The figure shows three views and two pictorial views of one solid part (mm, origin at its lowest corner). Answer the questions. A direction names the side the tool comes from. Round coordinates to 2 decimals unless told otherwise and drop trailing zeros. Order: outer loops, then holes, each group sorted by start corner. A loop starts at its lowest first (then second) coordinate and runs counter-clockwise, first axis right, second up. Notation, with made-up numbers: (33, -16.5) -> (75, -16.5) arc R20 ccw to (75, 17.5) -> close; hole circle Ø4 at (38.5, 22.5). An arc over 180 degrees is marked (long way). Answer as a JSON object with one key per item and string values. Group by question number.
Item 1: Given P1, Ø6.5, axis at x = 19.5, y = 6, coming from the -Z side; P2, Ø3, axis at x = 118, z = 2.5, coming from the +Y side; P3, Ø10, axis at x = 71.5, z = 26, coming from the +Y side; P4, Ø18, axis at x = 57, y = 71.5, coming from the -Z side, each flat-ended and moving along its own axis, determine where each tip first touches the part or whether it passes through.
Item 2: The mould has two halves that part along Y. Classify the marked faces 6, 7 and 8: pulls with the +Y half, pulls with the -Y half, needs draft (parallel to the pull), parting line crosses it, or undercut.
Item 3: For the marked faces 1, 2, 3, 4 and 5, determine the directions among +Z, -Z, +X, -X, +Y, -Y from which every point of the face is accessible in a straight line to the end or side of a thin tool.
Item 4: Section D-D, the plane z = 16.5 is taken. Write down the section's boundary in (x, y).
Item 5: Section C-C, the plane y = 12 is taken. Write down the section's boundary in (x, z), plus the area to 3 significant figures.
Item 6: Consider probe 1 along Y at (x, z) = (65, 6.5); probe 2 along Z at (x, y) = (88, 68); probe 3 along X at (y, z) = (72, 6). Determine where each line is inside the solid, lowest interval first. Write a range as from..to.
Item 7: Section A-A, the plane x = 65 is taken. Write down the section's boundary in (y, z).
Item 8: Section B-B, the plane z = 37 is taken. Write down the section's boundary in (x, y).
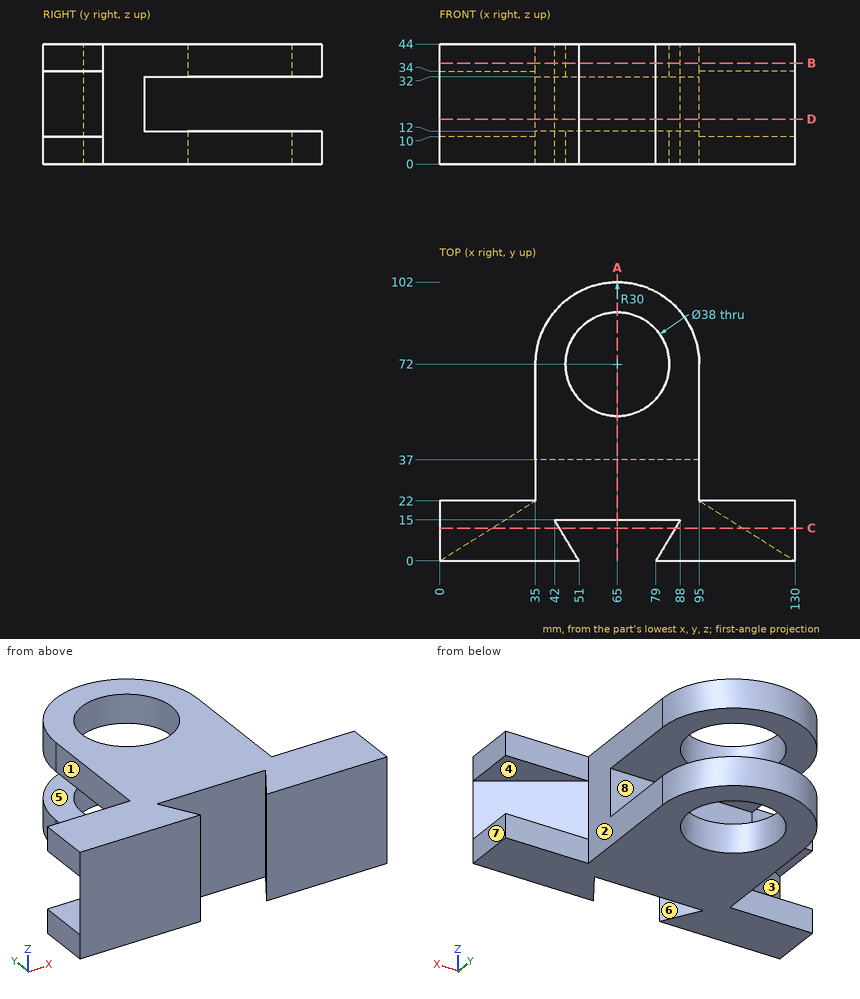
Values found:
{
 "1": {"P1": "z = 0", "P2": "y = 22", "P3": "y = 37", "P4": "through"},
 "2": {"face 6": "undercut", "face 7": "needs draft", "face 8": "pulls with the +Y half"},
 "3": {"face 1": "+Z, -Z, -X, +Y", "face 2": "+Z, -Z, +X, +Y", "face 3": "-X, +Y", "face 4": "+X, +Y", "face 5": "+X, -X, +Y"},
 "4": {"outline": "(0, 0) -> (51, 0) -> (42, 15) -> (88, 15) -> (79, 0) -> (130, 0) -> (95, 22) -> (95, 37) -> (35, 37) -> (35, 22) -> close"},
 "5": {"outline": "(0, 0) -> (43.8, 0) -> (43.8, 44) -> (0, 44) -> (0, 34) -> (19.09, 34) -> (19.09, 10) -> (0, 10) -> close; (86.2, 0) -> (130, 0) -> (130, 10) -> (110.91, 10) -> (110.91, 34) -> (130, 34) -> (130, 44) -> (86.2, 44) -> close", "area": "2,940 mm2"},
 "6": {"probe 1": "15..53, 91..102", "probe 2": "0..12, 32..44", "probe 3": "35..46, 84..95"},
 "7": {"outline": "(15, 0) -> (53, 0) -> (53, 12) -> (37, 12) -> (37, 32) -> (53, 32) -> (53, 44) -> (15, 44) -> close; (91, 0) -> (102, 0) -> (102, 12) -> (91, 12) -> close; (91, 32) -> (102, 32) -> (102, 44) -> (91, 44) -> close"},
 "8": {"outline": "(0, 0) -> (51, 0) -> (42, 15) -> (88, 15) -> (79, 0) -> (130, 0) -> (130, 22) -> (95, 22) -> (95, 72) arc R30 ccw to (35, 72) -> (35, 22) -> (0, 22) -> close; hole circle Ø38 at (65, 72)"}
}
